Job drawing, mm, ordinate dimensions from the low corner. One solid piece. Give positions to 0.01 mm unless a question says otherwise; leave off trailing zeros. Order: outer loops, then holes, each group sorted by start corner. A loop starts at its lowest first (then second) coordinate and runs counter-clockwise, first axis right, second up.
1. Slice it at D-D on x = 4. List the corners of the cut face in (y, z) (1 decimal).
2. Drop flat-ended pins along their axis: pin 1 Ø3 at (x, z) = (16, 11) entering from -Y; pin 2 Ø6 at (y, z) = (8, 3.5) entering from -X; pin 3 Ø1.5 at (x, y) = (24.5, 38) entering from -Z. Give the stop position or say it passes through.
3. Slice it at B-B on z = 7. List the corners of the cut face in (x, y).
4. Slice it at A-A on x = 43.5. List the corners of the cut face in (y, z) (1 decimal).
5. Mould opens along Y. For the marked faces 1, 2 and 3 say: +Y half, -Y half, draft (parallel to the pull), parting line (faces both ways), or undercut.
6. Slice it at C-C on y = 15. List the corners of the cut face in (x, z) (1 decimal), and give its area (3 significant figures).
7. Probe line 1 (Y direction, x = 47.5, z = 14.5); line 2 (X direction, y = 60, z = 12.5); line 3 (Z direction, x = 30.5, y = 54.5) (1 decimal). List the from-to ranges inside material, lowest first.
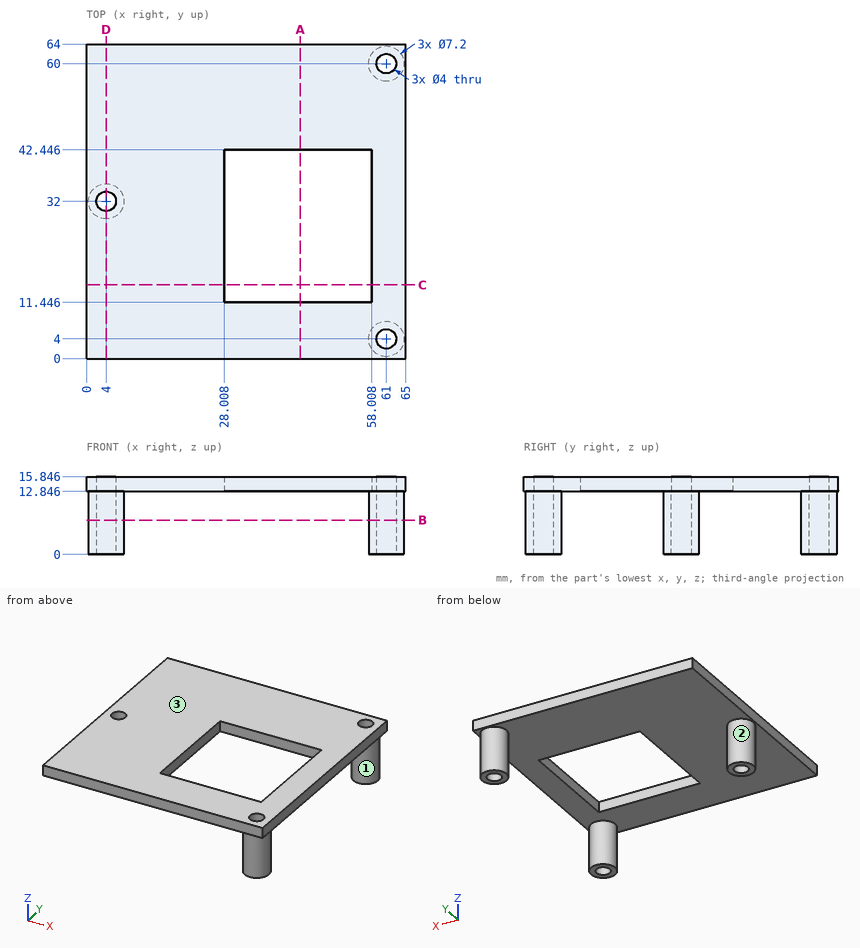
Data:
1. outline: (0, 12.8) - (28.4, 12.8) - (28.4, 0) - (30, 0) - (30, 15.8) - (0, 15.8) - close; (34, 0) - (35.6, 0) - (35.6, 12.8) - (64, 12.8) - (64, 15.8) - (34, 15.8) - close
2. pin 1: passes through
2. pin 2: stops at x = 57.54
2. pin 3: stops at z = 12.85
3. outline: circle Ø7.2 at (4, 32); circle Ø7.2 at (61, 4); circle Ø7.2 at (61, 60); hole circle Ø4 at (4, 32); hole circle Ø4 at (61, 4); hole circle Ø4 at (61, 60)
4. outline: (0, 12.8) - (11.4, 12.8) - (11.4, 15.8) - (0, 15.8) - close; (42.4, 12.8) - (64, 12.8) - (64, 15.8) - (42.4, 15.8) - close
5. face 1: undercut
5. face 2: parting line
5. face 3: draft
6. outline: (0, 12.8) - (28, 12.8) - (28, 15.8) - (0, 15.8) - close; (58, 12.8) - (65, 12.8) - (65, 15.8) - (58, 15.8) - close
6. area: 105 mm2
7. line 1: y = 0 to 11.45, 42.45 to 64
7. line 2: x = 57.4 to 59, 63 to 64.6
7. line 3: z = 12.8 to 15.8
